Could you check a few things on this model? Use its own coordinates, in mm. A direction names the side the tool comes from. Round coordinates to 2 decimals unless told otherwise and drop trailing zeros. Write each loop counter-clockwise with the first axis right and the second up, starting at its lowest first coordinate (ties: lowest second). Pieces come first, ordered by that corner, then holes. Notation, with made-up numbers: (-15, 16) -> (23, 16) arc R16 ccw to (23, 37) -> close; hole circle Ø2 at (17.5, 51). An arc over 180 degrees is marked (long way). Answer in a Markdown table with one row per item. Add a question column.
```python
from build123d import *

# Parameters (mm, degrees)
SKETCH_1_W          = 36
SKETCH_1_H          = 26
EXTRUDE_1_DEPTH     = 14.6
SKETCH_2_W          = 33
SKETCH_2_H          = 22
CUT_EXTRUDE_1_DEPTH = 13
SKETCH_3_W          = 36
SKETCH_3_H          = 26
CUT_EXTRUDE_2_DEPTH = 4.5
SKETCH_4_W          = 1.5
SKETCH_4_H          = 22
CUT_EXTRUDE_3_DEPTH = 6
SKETCH_7_W          = 17
SKETCH_7_H          = 2
SKETCH_7_W_2        = 1.5
SKETCH_7_H_2        = 22
EXTRUDE_4_DEPTH     = 3
SKETCH_5_W          = 4
SKETCH_5_H          = 3
EXTRUDE_5_DEPTH     = 2
SKETCH_8_W          = 4
SKETCH_8_H          = 26
EXTRUDE_6_DEPTH     = 2.5


with BuildPart() as part:
    # 草图1 → 凸台-拉伸1 (new body)
    with BuildSketch(Plane(origin=(0, 0, 0), x_dir=(1, 0, 0), z_dir=(0, 1, 0))):
        Rectangle(SKETCH_1_W, SKETCH_1_H)
    extrude(amount=EXTRUDE_1_DEPTH)

    # 草图2 → 切除-拉伸1 (cut)
    with BuildSketch(Plane(origin=(0, 14.6, 0), x_dir=(1, 0, 0), z_dir=(0, 1, 0))):
        Rectangle(SKETCH_2_W, SKETCH_2_H)
    extrude(amount=-CUT_EXTRUDE_1_DEPTH, mode=Mode.SUBTRACT)

    # 草图3 → 切除-拉伸2 (cut)
    with BuildSketch(Plane(origin=(0, 14.6, 0), x_dir=(1, 0, 0), z_dir=(0, 1, 0))):
        Rectangle(SKETCH_3_W, SKETCH_3_H)
    extrude(amount=-CUT_EXTRUDE_2_DEPTH, mode=Mode.SUBTRACT)

    # 草图4 → 切除-拉伸3 (cut)
    with BuildSketch(Plane(origin=(0, 10.1, 0), x_dir=(1, 0, 0), z_dir=(0, 1, 0))):
        with Locations((-17.25, 0)):
            Rectangle(SKETCH_4_W, SKETCH_4_H)
    extrude(amount=-CUT_EXTRUDE_3_DEPTH, mode=Mode.SUBTRACT)

    # 草图7 → 凸台-拉伸4 (add)
    with BuildSketch(Plane(origin=(0, 10.1, 0), x_dir=(1, 0, 0), z_dir=(0, 1, 0))):
        with Locations((-9.5, 12)):
            Rectangle(SKETCH_7_W, SKETCH_7_H)
        with Locations((-9.5, -12)):
            Rectangle(SKETCH_7_W, SKETCH_7_H)
        with Locations((17.25, 0)):
            Rectangle(SKETCH_7_W_2, SKETCH_7_H_2)
    extrude(amount=EXTRUDE_4_DEPTH)

    # 草图5 → 凸台-拉伸5 (add)
    with BuildSketch(Plane(origin=(0, 0, 0), x_dir=(-1, 0, 0), z_dir=(0, -1, 0))):
        with Locations((-12.2, -11.5)):
            Rectangle(SKETCH_5_W, SKETCH_5_H)
        with Locations((12.2, -11.5)):
            Rectangle(SKETCH_5_W, SKETCH_5_H)
        with Locations((-12.2, 11.5)):
            Rectangle(SKETCH_5_W, SKETCH_5_H)
        with Locations((12.2, 11.5)):
            Rectangle(SKETCH_5_W, SKETCH_5_H)
    extrude(amount=EXTRUDE_5_DEPTH)

    # 草图8 → 凸台-拉伸6 (add)
    with BuildSketch(Plane(origin=(0, -2, 0), x_dir=(-1, 0, 0), z_dir=(0, -1, 0))):
        with Locations((-12.2, 0)):
            Rectangle(SKETCH_8_W, SKETCH_8_H)
        with Locations((12.2, 0)):
            Rectangle(SKETCH_8_W, SKETCH_8_H)
    extrude(amount=EXTRUDE_6_DEPTH)


solid = part.part
```
(1) Suppose I cut it at B-B, the plane z = -5. Please give me the cut outline in (x, y).
(2) On a 3-axis mill with a long thin cutter (end or side, diameter ignored), from which of +Z, -Z, +X, -X, +Y, -Y can I reach the whole of each face in a straight line? I mean faces 4 (the face through (-14.2, -3, 0)), 5 (the face through (17, 13.1, 0)), 6 (the face through (-1, 7, -11)), 7 (the face through (-1, 12, -12)), 8 (the face through (-12, -2, 0)). Say none if no direction works.
(3) Suppose I cut it at A-A, the plane y = -3.25. Please give me the cut outline in (x, z), then the cut area to 3 significant figures.
(4) Suppose I cut it at D-D, the plane x = -12.5. Please give me the cut outline in (y, z), then the cut area to 3 significant figures.
(5) If we mould it in two halves opening along Z, with no side actions, what happens to faces 1 (the face through (16.5, 7, 0)), 2 (the face through (0, 4, -13)), 3 (the face through (18, 6, 0))? For each: pulls with the +Z half, pulls with the -Z half, needs draft (parallel to the pull), parting line crosses it, or undercut.
(6) Suppose I cut it at C-C, the plane y = 10.75. Please give me the cut outline in (x, z), then the cut area to 3 significant figures.
(7) I need wall thicknesses on L1, parallel to Z at x = 16, y = 4.5; L2, parallel to Y at x = 12.5, z = 1.25; L3, parallel to X at y = -3, z = -2.75. Which ranges of each line are inside material? Lowest first, please.
(8) For P1, Ø1.5, axis at x = -12, z = -4.5, coming from the +Y side; P2, Ø9, axis at y = 9.5, z = 3.5, coming from the -X side; P3, Ø2, axis at y = -2, z = -2.5, coming from the -X side, each with a flat end and sliding along its axis, tell me the tip position at first contact or that it passes through.
Response:
| question | item | result |
|---|---|---|
| 1 | outline | (-18, 0) -> (18, 0) -> (18, 13.1) -> (16.5, 13.1) -> (16.5, 1.6) -> (-16.5, 1.6) -> (-16.5, 4.1) -> (-18, 4.1) -> close; (-14.2, -4.5) -> (-10.2, -4.5) -> (-10.2, -2) -> (-14.2, -2) -> close; (10.2, -4.5) -> (14.2, -4.5) -> (14.2, -2) -> (10.2, -2) -> close |
| 2 | face 4 | +Z, -Z, -X, -Y |
| 2 | face 5 | +Z, -Z, +X, -X, +Y |
| 2 | face 6 | +Y |
| 2 | face 7 | +Z, -Z, +X, +Y |
| 2 | face 8 | +X, -X |
| 3 | outline | (-14.2, -13) -> (-10.2, -13) -> (-10.2, 13) -> (-14.2, 13) -> close; (10.2, -13) -> (14.2, -13) -> (14.2, 13) -> (10.2, 13) -> close |
| 3 | area | 208 mm² |
| 4 | outline | (-4.5, -13) -> (13.1, -13) -> (13.1, -11) -> (1.6, -11) -> (1.6, 11) -> (13.1, 11) -> (13.1, 13) -> (-4.5, 13) -> close; hole (-2, -10) -> (0, -10) -> (0, 10) -> (-2, 10) -> close |
| 4 | area | 165 mm² |
| 5 | face 1 | undercut |
| 5 | face 2 | pulls with the -Z half |
| 5 | face 3 | needs draft |
| 6 | outline | (-18, -13) -> (-1, -13) -> (-1, -11) -> (-18, -11) -> close; (-18, 11) -> (-1, 11) -> (-1, 13) -> (-18, 13) -> close; (16.5, -11) -> (18, -11) -> (18, 11) -> (16.5, 11) -> close |
| 6 | area | 101 mm² |
| 7 | L1 | -13 to -11, 11 to 13 |
| 7 | L2 | -4.5 to -2, 0 to 1.6 |
| 7 | L3 | -14.2 to -10.2, 10.2 to 14.2 |
| 8 | P1 | y = 1.6 |
| 8 | P2 | x = 16.5 |
| 8 | P3 | x = -14.2 |
